Check sheet for the modelled part. Datum: model origin and axes. Units: mm. Face numbers are marked on the shaded views. Round coordinates to 2 decimals unless told otherwise and drop trailing zeros. Write each loop counter-clockwise with the first axis right and the second up, starting at its lowest first coordinate (ties: lowest second). Pieces come first, ordered by that corner, then holes. Notation, with made-up numbers: (75.25, -37) -> (102.25, -37) arc R25 cw to (102.25, -6) -> close; hole circle Ø10 at (52.5, -5). An arc over 180 degrees is marked (long way). Write item = value, one per line.
from build123d import *

# Parameters (mm, degrees)
F2_R     = 2
F3_R     = 1
F4_R     = 2.15
F5_DEPTH = 0.3
F7_DEPTH = 0.5
F8_R     = 0.2
F9_SIZE  = 0.5


with BuildPart() as f1:
    # F0 (on Front) → F1 (revolve)
    with BuildSketch(Plane.XZ):
        Polygon((-1.9, -9.478535), (0, -9.478535), (0, 2.5), (-3.5, 2.5), (-6, 0), (-6, -2.5), (-1.9, -2.5), align=None)
    revolve(axis=Axis((0, 0, -3.489268), (0, 0, -1)))

    # F2
    f2_edges = [f1.edges().sort_by_distance(p)[0] for p in [
        (6, 0, 0),
    ]]
    fillet(f2_edges, radius=F2_R)

    # F3
    f3_edges = [f1.edges().sort_by_distance(p)[0] for p in [
        (6, 0, -2.5),
    ]]
    fillet(f3_edges, radius=F3_R)

    # F4 (on Right) → F5 (join, symmetric)
    with BuildSketch(Plane.YZ):
        with Locations((0, -7.328535)):
            Circle(F4_R)
    extrude(amount=F5_DEPTH, both=True)

    # F6 (on face) → F7 (cut)
    with BuildSketch(Plane.XY.offset(2.5)):
        Polygon((-1.035534, 2.5), (-2.5, 1.035534), (-2.5, -1.035534), (-1.035534, -2.5), (1.035534, -2.5), (2.5, -1.035534), (2.5, 1.035534), (1.035534, 2.5), align=None)
        Polygon((-2, -0.828427), (-2, 0.828427), (-0.828427, 2), (0.828427, 2), (2, 0.828427), (2, -0.828427), (0.828427, -2), (-0.828427, -2), align=None, mode=Mode.SUBTRACT)
    extrude(amount=-F7_DEPTH, mode=Mode.SUBTRACT)

    # F8
    f8_edges = [f1.edges().sort_by_distance(p)[0] for p in [
        (-1.767767, 1.767767, 2),
        (-2.5, 0, 2),
        (-1.767767, -1.767767, 2),
        (0, -2.5, 2),
        (1.767767, -1.767767, 2),
        (2.5, 0, 2),
        (1.767767, 1.767767, 2),
        (0, 2.5, 2),
        (0, -2, 2),
        (-1.414214, -1.414214, 2),
        (-2, 0, 2),
        (-1.414214, 1.414214, 2),
        (0, 2, 2),
        (1.414214, 1.414214, 2),
        (2, 0, 2),
        (1.414214, -1.414214, 2),
    ]]
    fillet(f8_edges, radius=F8_R)

    # F9
    f9_edges = [f1.edges().sort_by_distance(p)[0] for p in [
        (1.9, 0, -9.478535),
    ]]
    chamfer(f9_edges, length=F9_SIZE)


solid = f1.part
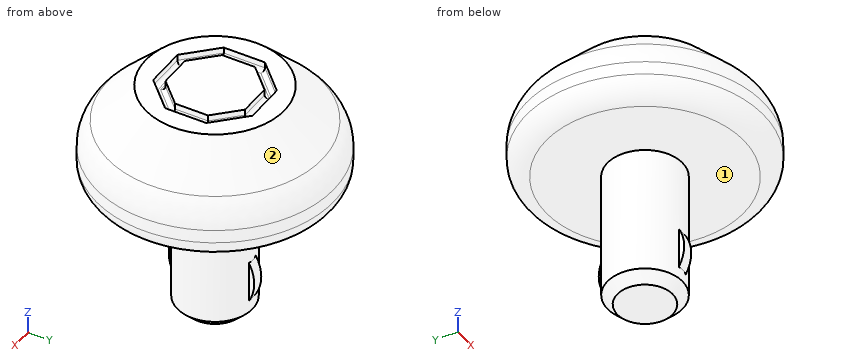
(1) Go/stop test with flat-tipped pins: P1, Ø5, axis at x = 4.5, z = 1, coming from the -Y side; P2, Ø1.5, axis at x = 4.5, z = -6, coming from the -Y side; P3, Ø2, axis at x = 3.5, z = -0.5, coming from the +Y side; P4, Ø5, axis at x = 3.5, y = -5, coming from the -Z side. Record where each tip stops, or that it passes through.
Worked answers:
P1 = -5.44
P2 = through
P3 = 5.44
P4 = -2.5
(2) Material ranges on L1, parallel to Z at x = -1.25, y = -2; L2, parallel to Z at x = 3.25, y = 3.25; L3, parallel to Y at x = 0, z = -3.75, recorded low to high. Write a range as [from, to].
Worked answers:
L1 = [-2.5, 2]
L2 = [-2.5, 1.4]
L3 = [-1.9, 1.9]
(3) Sectioned sample at A-A on z = -5.5. Enter the section's corners in (x, y).
Worked answers:
outline = circle Ø3.8 at (0, 0)
(4) Release check for a two-part mould opening along X. For the marked faces 1 and 2 record: pulls with the +X half, pulls with the -X half, needs draft (parallel to the pull), parting line crosses it, or undercut.
Worked answers:
face_1 = needs draft
face_2 = parting line crosses it
